Could you check a few things on this model? Use its own coordinates, in mm. Face numbers are marked on the shaded views. Coordinates: 2 decimals unless noted, no trailing zeros. Order: outer loops, then holes, each group sorted by start corner. A loop starts at its lowest first (then second) coordinate and runs counter-clockwise, first axis right, second up. Notation, with made-up numbers: (-32, 44.25) - (-24, 44.25) arc R29 ccw to (-24, 78.25) - close; hole circle Ø6 at (0.25, 65.25). An arc over 180 degrees is marked (long way). Answer as a JSON object with one key per item and string values. Group by question number.
(1) Imagine slicing it at C-C, the plane z = 8.5. Write out the boundary of the cut face in (x, y).
(2) Imagine slicing it at D-D, the plane y = 8.5. Write out the boundary of the cut face in (x, z), and give its area (3 significant figures).
(3) We'd pull the mould along Y, two halves only. Please class the marked faces 1, 2 and 3: pulls with the +Y half, pulls with the -Y half, needs draft (parallel to the pull), parting line crosses it, or undercut.
(4) Imagine slicing it at A-A, the plane x = -34. Write out the boundary of the cut face in (y, z), and give its area (3 significant figures).
(5) Please list where these lines run through material, in increasing order: probe 1 along Y at (x, z) = (-16, 35); probe 2 along Z at (x, y) = (-7.5, 15.5); probe 3 along Z at (x, y) = (-33.5, 20).
(6) Imagine slicing it at B-B, the plane y = 24. Write out the boundary of the cut face in (x, z), and give its area (3 significant figures).
(7) Will these pins go through, and if not, where does the flat tip stop? P1, Ø1.6, axis at x = -25.5, y = 0.5, coming from the +Z side; P2, Ø2, axis at x = -0.5, y = 26, coming from the +Z side; P3, Ø0.5, axis at y = 15.5, z = 50.5, coming from the -X side.
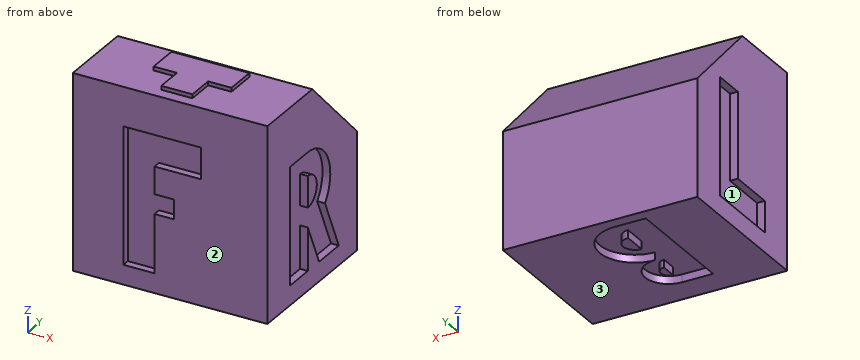
from build123d import *

# Parameters (mm, degrees)
F0_W      = 50
F0_H      = 50
F1_DEPTH  = 40
F2_SIZE   = 20
F4_DEPTH  = 2
F6_DEPTH  = 2
F8_DEPTH  = 2
F10_DEPTH = 1
F12_DEPTH = 2


with BuildPart() as f1:
    # F0 (on Front) → F1 (new body)
    with BuildSketch(Plane.XZ):
        with Locations((-25, 25)):
            Rectangle(F0_W, F0_H)
    extrude(amount=-F1_DEPTH)

    # F2
    f2_edges = [f1.edges().sort_by_distance(p)[0] for p in [
        (-25, 40, 50),
    ]]
    chamfer(f2_edges, length=F2_SIZE)

    # F3 (on face) → F4 (cut)
    with BuildSketch(Plane.XZ):
        Polygon((-37, 40), (-37, 5), (-29, 5), (-29, 20), (-24, 20), (-24, 25), (-29, 25), (-29, 32), (-17, 32), (-17, 40), align=None)
    extrude(amount=-F4_DEPTH, mode=Mode.SUBTRACT)

    # F5 (on face) → F6 (cut)
    with BuildSketch(Plane.YZ):
        with BuildLine():
            Line((10, 35), (10, 5))
            Line((10, 5), (18, 5))
            Line((18, 5), (18, 16))
            Line((18, 16), (23, 5))
            Line((23, 5), (31.78767, 5))
            Line((31.78767, 5), (25.633212, 18.539808))
            ThreePointArc((25.633212, 18.539808), (27.071988, 29.207023), (18, 35))
            Line((18, 35), (10, 35))
        make_face()
        with BuildLine():
            Line((18, 21), (18, 29))
            ThreePointArc((18, 29), (22, 25), (18, 21))
        make_face(mode=Mode.SUBTRACT)
    extrude(amount=-F6_DEPTH, mode=Mode.SUBTRACT)

    # F7 (on face) → F8 (cut)
    with BuildSketch(Plane(origin=(-50, 0, 0), x_dir=(0, -1, 0), z_dir=(-1, 0, 0))):
        Polygon((-22, 35), (-30, 35), (-30, 5), (-10, 5), (-10, 13), (-22, 13), align=None)
    extrude(amount=-F8_DEPTH, mode=Mode.SUBTRACT)

    # F9 (on face) → F10 (join)
    with BuildSketch(Plane.XY.offset(50)):
        Polygon((-29, 10), (-29, 3), (-21, 3), (-21, 10), (-15, 10), (-15, 18), (-35, 18), (-35, 10), align=None)
    extrude(amount=F10_DEPTH)

    # F11 (on face) → F12 (cut)
    with BuildSketch(Plane(origin=(0, 0, 0), x_dir=(1, 0, 0), z_dir=(0, 0, -1))):
        with BuildLine():
            Line((-35, -7), (-35, -37))
            Line((-35, -37), (-27, -37))
            ThreePointArc((-27, -37), (-18, -28), (-27, -19))
            ThreePointArc((-27, -19), (-21, -13), (-27, -7))
            Line((-27, -7), (-35, -7))
        make_face()
        with BuildLine():
            ThreePointArc((-27, -25), (-24, -28), (-27, -31))
            Line((-27, -31), (-27, -25))
        make_face(mode=Mode.SUBTRACT)
        with BuildLine():
            Line((-27, -15), (-27, -11))
            ThreePointArc((-27, -11), (-25, -13), (-27, -15))
        make_face(mode=Mode.SUBTRACT)
    extrude(amount=-F12_DEPTH, mode=Mode.SUBTRACT)


solid = f1.part
Result set:
{
 "1": {"outline": "(-50, 0) - (-37, 0) - (-37, 2) - (-29, 2) - (-29, 0) - (0, 0) - (0, 10) - (-2, 10) - (-2, 18) - (0, 18) - (0, 21.41) - (-2, 21.41) - (-2, 30.2) - (0, 30.2) - (0, 40) - (-50, 40) - (-50, 30) - (-48, 30) - (-48, 10) - (-50, 10) - close"},
 "2": {"outline": "(-50, 0) - (-35, 0) - (-35, 2) - (-23.03, 2) - (-23.03, 0) - (0, 0) - (0, 50) - (-21, 50) - (-21, 51) - (-29, 51) - (-29, 50) - (-50, 50) - close", "area": "2,480 mm^2"},
 "3": {"face 1": "undercut", "face 2": "pulls with the -Y half", "face 3": "needs draft"},
 "4": {"outline": "(0, 0) - (7, 0) - (7, 2) - (37, 2) - (37, 0) - (40, 0) - (40, 30) - (20, 50) - (18, 50) - (18, 51) - (10, 51) - (10, 50) - (0, 50) - (0, 40) - (2, 40) - (2, 5) - (0, 5) - close", "area": "1,680 mm^2"},
 "5": {"probe 1": "y = 0 to 35", "probe 2": "z = 0 to 50", "probe 3": "z = 2 to 50"},
 "6": {"outline": "(-50, 0) - (-35, 0) - (-35, 2) - (-18.94, 2) - (-18.94, 0) - (0, 0) - (0, 5) - (-2, 5) - (-2, 33) - (0, 33) - (0, 46) - (-50, 46) - (-50, 35) - (-48, 35) - (-48, 5) - (-50, 5) - close", "area": "2,150 mm^2"},
 "7": {"P1": "stops at z = 50", "P2": "stops at z = 45", "P3": "stops at x = -35"}
}
